Geometry check sheet. Reference: drawing and pictorial views, mm from the part's lowest x, y, z. A direction names the side the tool comes from. Give positions to 0.01 mm unless a question says otherwise; leave off trailing zeros. Order: outer loops, then holes, each group sorted by start corner. A loop starts at its lowest first (then second) coordinate and runs counter-clockwise, first axis right, second up. Notation, with made-up numbers: (7.25, 1) -> (33.25, 1) arc R31 ccw to (33.25, 38) -> close; hole circle Ø7 at (-4, 65). An arc over 180 degrees is marked (long way). Write each question's results on one line, items separated by ' | '. Start each with the question number.
1. Cross-section at B-B, the plane y = 64. Enter the section's corners in (x, z).
2. Material ranges on L1, parallel to X at y = 30, z = 64; L2, parallel to Y at x = 89, z = 65; L3, parallel to Z at x = 71.5, y = 73, recorded low to high. Write a range as from..to.
3. Cross-section at C-C, the plane x = 57. Enter the section's corners in (y, z) (1 decimal), then the cut area to 3 significant figures.
4. Cross-section at A-A, the plane x = 28.5. Enter the section's corners in (y, z) (1 decimal), then the cut area to 3 significant figures.
5. Set-up check for the marked faces 1, 2, 3 and 4: record each of +Z, -Z, +X, -X, +Y, -Y from which the full face is reachable in a straight line by a thin tool's end or side.
6. Cross-section at D-D, the plane z = 11. Enter the section's corners in (x, y), then the cut area to 3 significant figures.
7. Mould release check, pull along Y, two halves, no side actions. Record for the marked faces 5, 6 and 7: +Y half, -Y half, draft (parallel to the pull), parting line (faces both ways), or undercut.
8. Depth check by flat-ended pin: pin 1 Ø7.5 at (y, z) = (91.5, 63) entering from -X; pin 2 Ø8 at (x, y) = (89.9, 87.44) entering from -Z; pin 3 Ø2.5 at (y, z) = (94, 67) entering from +X; pin 4 Ø1 at (x, y) = (91.5, 80.5) entering from -Z. Enter the tip coordinate at first touch or a pass-through.
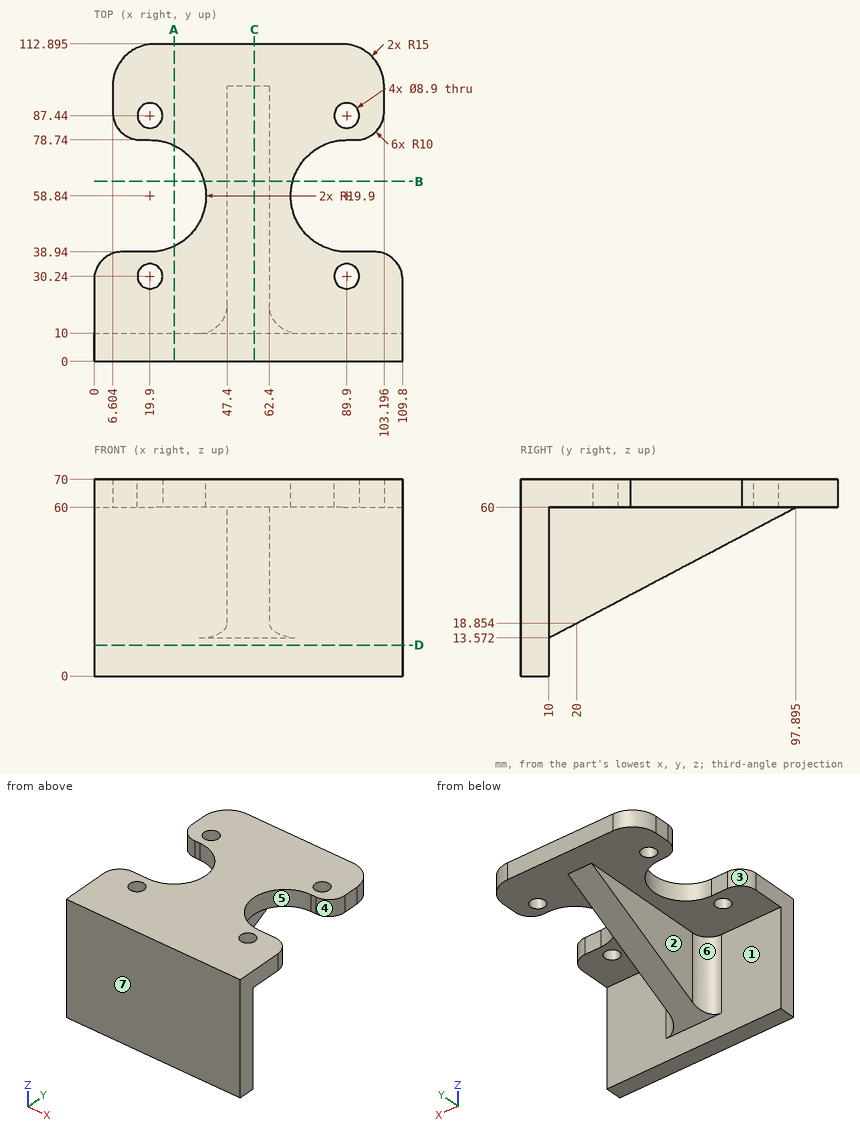
Results below:
1) outline: (39.12, 60) -> (47.4, 60) -> (47.4, 42.1) -> (62.4, 42.1) -> (62.4, 60) -> (70.68, 60) -> (70.68, 70) -> (39.12, 70) -> close
2) L1: x = 0.06..15.46, 24.34..85.46, 94.34..109.74 | L2: y = 0..25.88, 34.6..38.96, 78.72..83.08, 91.8..112.87 | L3: z = 60..70
3) outline: (0, 0) -> (10, 0) -> (10, 13.6) -> (97.9, 60) -> (112.9, 60) -> (112.9, 70) -> (0, 70) -> close | area: 3,770 mm²
4) outline: (0, 0) -> (10, 0) -> (10, 60) -> (40.9, 60) -> (40.9, 70) -> (0, 70) -> close; (76.8, 60) -> (112.9, 60) -> (112.9, 70) -> (76.8, 70) -> close | area: 1,370 mm²
5) face 1: -Z, +Y | face 2: -Z, -X, +Y | face 3: +Z, -Z, -X | face 4: +Z, -Z, +X
6) outline: (0, 0) -> (109.8, 0) -> (109.8, 10) -> (0, 10) -> close | area: 1,100 mm²
7) face 5: undercut | face 6: +Y half | face 7: -Y half
8) pin 1: stops at x = 6.6 | pin 2: passes through | pin 3: stops at x = 103.2 | pin 4: stops at z = 60
